Source: CAD feature listing. Evaluate the final solid. Frame: model axes, mm. Coordinates: 2 decimals unless noted, no trailing zeros. Write each loop counter-clockwise with the first axis right and the second up, starting at its lowest first coordinate (ties: lowest second). Pieces come first, ordered by that corner, then holes. Notation, with made-up numbers: (17, -7.75) - (26, -7.75) arc R31 cw to (26, 20.25) - close; hole circle Ø1 at (-11, -12). An arc over 180 degrees is marked (long way). One line per question, with ' | ' between items. Start each with the question number.
Q1. Cut plane A-A, the plane z = 254. Return loops of the section in (x, y), plus the area to 3 significant figures.
Q2. Contact query for flat-ended pins moving along their axis: P1, Ø7.5, axis at x = 101.6, z = 254, coming from the +Y side; P2, Ø0.8, axis at y = -0.5, z = 131, coming from the +X side. Output: stop coordinate, or through.
Q3. Line query: line 1 (Z direction, x = 101.6, y = -1.2); line 2 (X direction, y = -1, z = 105); line 3 (X direction, y = -1.2, z = 184.5). Output: solid intervals per line, ascending.
Q4. Cut plane B-B, the plane y = -0.35. Return loops of the section in (x, z), plus the area to 3 significant figures.
Q5. Cut plane C-C, the plane x = 101.6. Return loops of the section in (y, z).
Q6. Cut plane D-D, the plane z = 107.5. Return loops of the section in (x, y).
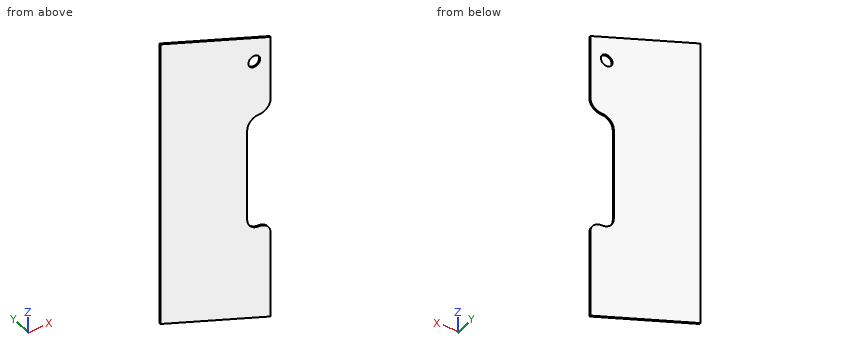
```python
from build123d import *

# Parameters (mm, degrees)
F0_R     = 6.35
F1_DEPTH = 1.5875


with BuildPart() as f1:
    # F0 (on Front) → F1 (new body)
    with BuildSketch(Plane.XZ):
        with BuildLine():
            Line((0, 317.5), (0, 0))
            Line((0, 0), (119.340963, -43.436558))
            Line((119.340963, -43.436558), (119.340963, 51.813442))
            ThreePointArc((119.340963, 51.813442), (115.621219, 60.793698), (106.640963, 64.513442))
            ThreePointArc((106.640963, 64.513442), (97.660707, 68.233186), (93.940963, 77.213442))
            Line((93.940963, 77.213442), (93.940963, 178.813442))
            ThreePointArc((93.940963, 178.813442), (97.660707, 187.793698), (106.640963, 191.513442))
            ThreePointArc((106.640963, 191.513442), (115.621219, 195.233186), (119.340963, 204.213442))
            Line((119.340963, 204.213442), (119.340963, 274.063442))
            Line((119.340963, 274.063442), (0, 317.5))
        make_face()
        with Locations((101.6, 254)):
            Circle(F0_R, mode=Mode.SUBTRACT)
    extrude(amount=F1_DEPTH)


solid = f1.part
```
Reply:
1) outline: (0, -1.59) - (95.25, -1.59) - (95.25, 0) - (0, 0) - close; (107.95, -1.59) - (119.34, -1.59) - (119.34, 0) - (107.95, 0) - close | area: 169 mm^2
2) P1: passes through | P2: stops at x = 93.94
3) line 1: z = -36.98 to 65.56, 190.47 to 247.65, 260.35 to 280.52 | line 2: x = 0 to 93.94 | line 3: x = 0 to 95.29
4) outline: (0, 0) - (119.34, -43.44) - (119.34, 51.81) arc R12.7 ccw to (106.64, 64.51) arc R12.7 cw to (93.94, 77.21) - (93.94, 178.81) arc R12.7 cw to (106.64, 191.51) arc R12.7 ccw to (119.34, 204.21) - (119.34, 274.06) - (0, 317.5) - close; hole circle Ø12.7 at (101.6, 254) | area: 34,500 mm^2
5) outline: (-1.59, -36.98) - (0, -36.98) - (0, 65.56) - (-1.59, 65.56) - close; (-1.59, 190.47) - (0, 190.47) - (0, 247.65) - (-1.59, 247.65) - close; (-1.59, 260.35) - (0, 260.35) - (0, 280.52) - (-1.59, 280.52) - close
6) outline: (0, -1.59) - (93.94, -1.59) - (93.94, 0) - (0, 0) - close
